Could you check a few things on this model? Use its own coordinates, in mm. Give positions to 0.01 mm unless a question says otherwise; leave off trailing zeros. Order: outer loops, then holes, each group sorted by start corner. A loop starts at its lowest first (then second) coordinate and runs counter-clockwise, first axis right, second up. Notation, with made-up numbers: (67, 28) - (115, 28) arc R18 cw to (115, 38) - close; hole circle Ø8 at (-34.5, -35.5). An arc over 180 degrees is marked (long way). Put each result on its own line as item: value.
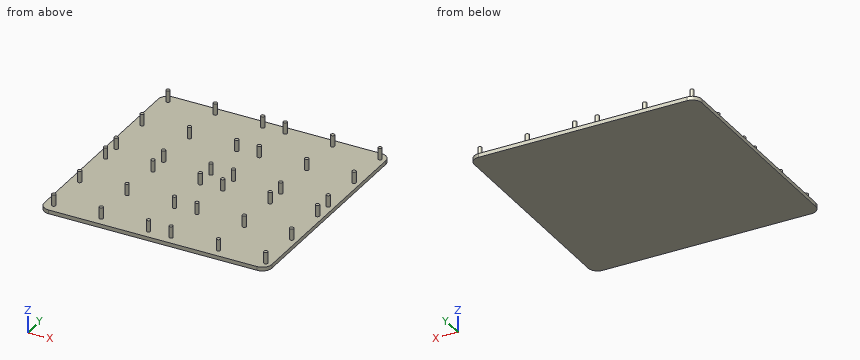
from build123d import *

# Parameters (mm, degrees)
F0_W     = 120
F0_H     = 120
F1_DEPTH = 2
F2_R     = 5
F3_R     = 1
F4_DEPTH = 6


with BuildPart() as f1:
    # F0 (on Top) → F1 (new body)
    with BuildSketch(Plane.XY):
        with Locations((-0.924264, -0.147626)):
            Rectangle(F0_W, F0_H)
    extrude(amount=F1_DEPTH)

    # F2
    f2_edges = [f1.edges().sort_by_distance(p)[0] for p in [
        (59.075736, -60.147626, 1),
        (59.075736, 59.852374, 1),
        (-60.924264, 59.852374, 1),
        (-60.924264, -60.147626, 1),
    ]]
    fillet(f2_edges, radius=F2_R)

    # F3 (on face) → F4 (join)
    with BuildSketch(Plane.XY.offset(2)):
        with Locations((-55.924264, -55.147626)):
            Circle(F3_R)
        with Locations((-55.924264, -30.147626)):
            Circle(F3_R)
        with Locations((-30.924264, -55.147626)):
            Circle(F3_R)
        with Locations((-30.924264, -30.147626)):
            Circle(F3_R)
        with Locations((-5.924264, -55.147626)):
            Circle(F3_R)
        with Locations((-5.924264, -30.147626)):
            Circle(F3_R)
        with Locations((-55.924264, -5.147626)):
            Circle(F3_R)
        with Locations((-30.924264, -5.147626)):
            Circle(F3_R)
        with Locations((-5.924264, -5.147626)):
            Circle(F3_R)
        with Locations((5.924264, -30.147626)):
            Circle(F3_R)
        with Locations((5.924264, -55.147626)):
            Circle(F3_R)
        with Locations((5.924264, -5.147626)):
            Circle(F3_R)
        with Locations((30.924264, -5.147626)):
            Circle(F3_R)
        with Locations((55.924264, -5.147626)):
            Circle(F3_R)
        with Locations((55.924264, -30.147626)):
            Circle(F3_R)
        with Locations((55.924264, -55.147626)):
            Circle(F3_R)
        with Locations((30.924264, -55.147626)):
            Circle(F3_R)
        with Locations((30.924264, -30.147626)):
            Circle(F3_R)
        with Locations((-55.924264, 5.147626)):
            Circle(F3_R)
        with Locations((-30.924264, 5.147626)):
            Circle(F3_R)
        with Locations((-5.924264, 5.147626)):
            Circle(F3_R)
        with Locations((5.924264, 5.147626)):
            Circle(F3_R)
        with Locations((30.924264, 5.147626)):
            Circle(F3_R)
        with Locations((55.924264, 5.147626)):
            Circle(F3_R)
        with Locations((-55.924264, 30.147626)):
            Circle(F3_R)
        with Locations((-30.924264, 30.147626)):
            Circle(F3_R)
        with Locations((5.924264, 30.147626)):
            Circle(F3_R)
        with Locations((-5.924264, 30.147626)):
            Circle(F3_R)
        with Locations((30.924264, 30.147626)):
            Circle(F3_R)
        with Locations((55.924264, 30.147626)):
            Circle(F3_R)
        with Locations((55.924264, 55.147626)):
            Circle(F3_R)
        with Locations((5.924264, 55.147626)):
            Circle(F3_R)
        with Locations((-5.924264, 55.147626)):
            Circle(F3_R)
        with Locations((-30.924264, 55.147626)):
            Circle(F3_R)
        with Locations((-55.924264, 55.147626)):
            Circle(F3_R)
        with Locations((30.924264, 55.147626)):
            Circle(F3_R)
    extrude(amount=F4_DEPTH)


solid = f1.part
1) I'm going to push a flat-ended pin straight in: pin 1 (10 mm diameter, centred on x = -8, y = -36, fed in from +Z). Where does the tip first touch, or does it pass through?
Filled in:
pin 1: stops at z = 2
2) Suppose I cut it at A-A, the plane x = -9. List the corners of the cut face in (y, z) for me, and give its area (3 significant figures).
Filled in:
outline: (-60.15, 0) - (59.85, 0) - (59.85, 2) - (-60.15, 2) - close
area: 240 mm^2
3) Suppose I cut it at C-C, the plane z = 5. State how many separate pieces and enclosed holes the cut face has, and give its area (3 significant figures).
Filled in:
separate pieces: 36
enclosed holes: 0
area: 113 mm^2
4) Suppose I cut it at B-B, the plane y = -18. List the corners of the cut face in (x, z) for me, and give its area (3 significant figures).
Filled in:
outline: (-60.92, 0) - (59.08, 0) - (59.08, 2) - (-60.92, 2) - close
area: 240 mm^2
5) If I drill on line 1 (X direction, y = 54.5, z = 7); line 2 (Z direction, x = -3, y = -20); line 3 (Y direction, x = 30.5, z = 4.5), over which ranges is the centre line in solid material (lowest first)? Write a range as [from, to].
Filled in:
line 1: x = [-56.69, -55.16], [-31.69, -30.16], [-6.69, -5.16], [5.16, 6.69], [30.16, 31.69], [55.16, 56.69]
line 2: z = [0, 2]
line 3: y = [-56.05, -54.24], [-31.05, -29.24], [-6.05, -4.24], [4.24, 6.05], [29.24, 31.05], [54.24, 56.05]
